Here's the drawing with two shaded views (mm, measured from the low corner). I have some questions. A direction names the side the tool comes from. Coordinates: 2 decimals unless noted, no trailing zeros. Loops run counter-clockwise (first coordinate to the right, second up) from the corner with the lowest first, then second, coordinate; pieces in that order, holes last. Notation, with made-up numbers: (-12.5, 15.25) - (7.5, 15.25) arc R17 cw to (7.5, 31.25) - close; hole circle Ø4 at (6, 17.25). An arc over 180 degrees is marked (long way). Use a Markdown table: item, result.
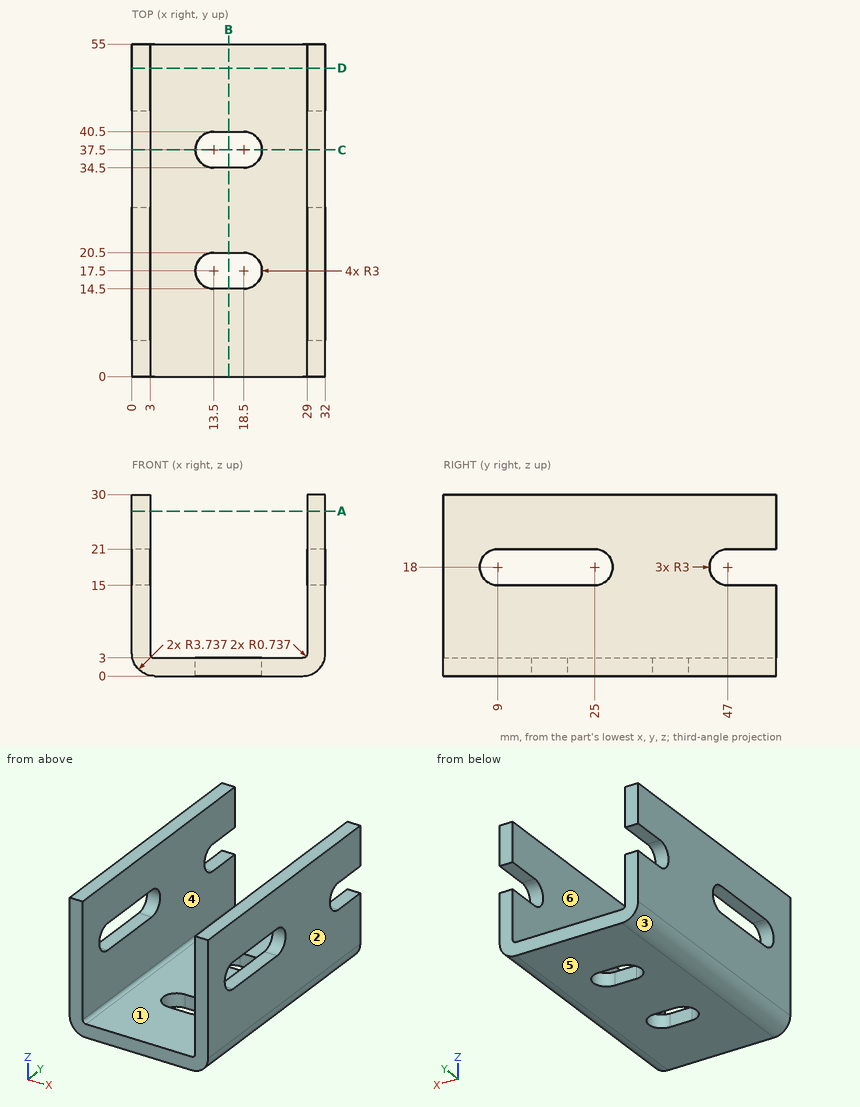
Q1. Will these pins go through, and if not, where does the flat tip stop? P1, Ø6, axis at x = 25, z = 11, coming from the +Y side; P2, Ø0.9, axis at x = 1, y = 50, coming from the -Z side; P3, Ø4, axis at x = 8.5, y = 10.5, coming from the +Z side; P4, Ø0.9, axis at x = 1.5, y = 13, coming from the -Z side (1 decimal).
Check values:
| item | result |
|---|---|
| P1 | through |
| P2 | z = 0.78 |
| P3 | z = 3 |
| P4 | z = 0.5 |
Q2. I want a section at B-B, the plane x = 16. Write out the boundary of the cut face in (y, z), then the cut area to 3 significant figures.
Check values:
| item | result |
|---|---|
| outline | (0, 0) - (14.5, 0) - (14.5, 3) - (0, 3) - close; (20.5, 0) - (34.5, 0) - (34.5, 3) - (20.5, 3) - close; (40.5, 0) - (55, 0) - (55, 3) - (40.5, 3) - close |
| area | 129 mm^2 |
Q3. I want a section at C-C, the plane y = 37.5. Write out the boundary of the cut face in (x, z), then the cut area to 3 significant figures.
Check values:
| item | result |
|---|---|
| outline | (0, 3.74) arc R3.74 ccw to (3.74, 0) - (10.5, 0) - (10.5, 3) - (3.74, 3) arc R0.74 cw to (3, 3.74) - (3, 30) - (0, 30) - close; (21.5, 0) - (28.26, 0) arc R3.74 ccw to (32, 3.74) - (32, 30) - (29, 30) - (29, 3.74) arc R0.74 cw to (28.26, 3) - (21.5, 3) - close |
| area | 219 mm^2 |
Q4. I want a section at D-D, the plane y = 51. Write out the boundary of the cut face in (x, z).
Check values:
| item | result |
|---|---|
| outline | (0, 3.74) arc R3.74 ccw to (3.74, 0) - (28.26, 0) arc R3.74 ccw to (32, 3.74) - (32, 15) - (29, 15) - (29, 3.74) arc R0.74 cw to (28.26, 3) - (3.74, 3) arc R0.74 cw to (3, 3.74) - (3, 15) - (0, 15) - close; (0, 21) - (3, 21) - (3, 30) - (0, 30) - close; (29, 21) - (32, 21) - (32, 30) - (29, 30) - close |
Q5. Which directions (+Z, -Z, +X, -X, +Y, -Y) give clear straight access to the entire face, cutting with the end or side of a thin tool? Please do the marked faces 1 and 2.
Check values:
| item | result |
|---|---|
| face 1 | +Z, +Y, -Y |
| face 2 | +Z, -Z, +X, +Y, -Y |
Q6. If we mould it in two halves opening along X, with no side actions, what happens to the marked faces 3, 4, 5 and 6? For each: pulls with the +X half, pulls with the -X half, needs draft (parallel to the pull), parting line crosses it, or undercut.
Check values:
| item | result |
|---|---|
| face 3 | pulls with the -X half |
| face 4 | undercut |
| face 5 | needs draft |
| face 6 | undercut |
Q7. Please list where these lines run through material, in increasing order: L1, parallel to X at y = 41, z = 24.5; L2, parallel to Z at x = 14.5, y = 42. Write a range as from..to.
Check values:
| item | result |
|---|---|
| L1 | 0..3, 29..32 |
| L2 | 0..3 |
Q8. I want a section at A-A, the plane z = 27.25. Write out the boundary of the cut face in (x, y), then the cut area to 3 significant figures.
Check values:
| item | result |
|---|---|
| outline | (0, 0) - (3, 0) - (3, 55) - (0, 55) - close; (29, 0) - (32, 0) - (32, 55) - (29, 55) - close |
| area | 330 mm^2 |
